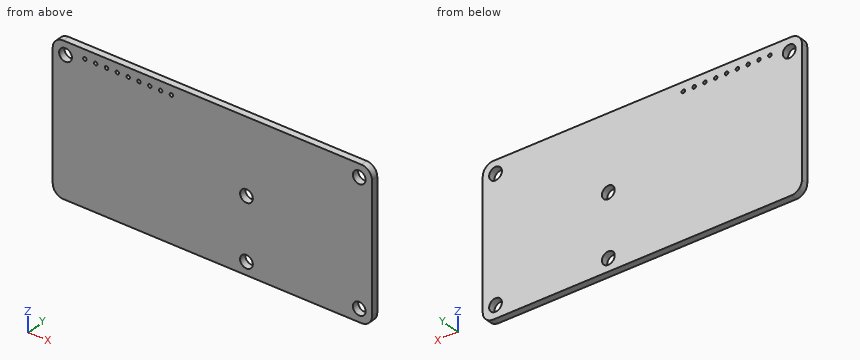
```python
from build123d import *

# Parameters (mm, degrees)
BOSS_EXTRUDE1_DEPTH = 1.6
SKETCH2_R           = 1.5
SKETCH2_R_2         = 0.406594982
CUT_EXTRUDE1_DEPTH  = 42.413282893


with BuildPart() as part:
    # Sketch1 → Boss-Extrude1 (new body)
    with BuildSketch(Plane(origin=(0, 0, 0), x_dir=(1, 0, 0), z_dir=(0, 1, 0))):
        with BuildLine():
            Line((-35, 17.5), (35, 17.5))
            ThreePointArc((35, 17.5), (36.767766953, 16.767766953), (37.5, 15))
            Line((37.5, 15), (37.5, -15))
            ThreePointArc((37.5, -15), (36.767766953, -16.767766953), (35, -17.5))
            Line((35, -17.5), (-35, -17.5))
            ThreePointArc((-35, -17.5), (-36.767766953, -16.767766953), (-37.5, -15))
            Line((-37.5, -15), (-37.5, 15))
            ThreePointArc((-37.5, 15), (-36.767766953, 16.767766953), (-35, 17.5))
        make_face()
    extrude(amount=BOSS_EXTRUDE1_DEPTH)

    # Sketch2 → Cut-Extrude1 (cut, through all)
    with BuildSketch(Plane(origin=(0, 1.6, 0), x_dir=(1, 0, 0), z_dir=(0, 1, 0))):
        with Locations(Location((-34.5, -14.5, 0), (0, 0, 270))):
            Circle(SKETCH2_R)
        with Locations(Location((34.5, -14.5, 0), (0, 0, 270))):
            Circle(SKETCH2_R)
        with Locations(Location((34.5, 14.5, 0), (0, 0, 270))):
            Circle(SKETCH2_R)
        with Locations(Location((8, 0, 0), (0, 0, 270))):
            Circle(SKETCH2_R)
        with Locations(Location((8, 14.5, 0), (0, 0, 270))):
            Circle(SKETCH2_R)
        with Locations(Location((-29.94018139, -15.399310559, 0), (0, 0, 270))):
            Circle(SKETCH2_R_2)
        with Locations(Location((-27.40018139, -15.399310559, 0), (0, 0, 270))):
            Circle(SKETCH2_R_2)
        with Locations(Location((-24.86018139, -15.399310559, 0), (0, 0, 270))):
            Circle(SKETCH2_R_2)
        with Locations(Location((-22.32018139, -15.399310559, 0), (0, 0, 270))):
            Circle(SKETCH2_R_2)
        with Locations(Location((-19.78018139, -15.399310559, 0), (0, 0, 270))):
            Circle(SKETCH2_R_2)
        with Locations(Location((-17.24018139, -15.399310559, 0), (0, 0, 270))):
            Circle(SKETCH2_R_2)
        with Locations(Location((-14.70018139, -15.399310559, 0), (0, 0, 270))):
            Circle(SKETCH2_R_2)
        with Locations(Location((-12.16018139, -15.399310559, 0), (0, 0, 270))):
            Circle(SKETCH2_R_2)
        with Locations(Location((-9.62018139, -15.399310559, 0), (0, 0, 270))):
            Circle(SKETCH2_R_2)
    extrude(amount=-CUT_EXTRUDE1_DEPTH, mode=Mode.SUBTRACT)


solid = part.part
```
Design review of the part built by this model. Coordinates are the model's own, in mm. Coordinates: 2 decimals unless noted, no trailing zeros. Order: outer loops, then holes, each group sorted by start corner. A loop starts at its lowest first (then second) coordinate and runs counter-clockwise, first axis right, second up. Notation, with made-up numbers: M -3.5,47 L 1.5,47 A12 ccw 1.5,69 Z; hole C 49.5,31.5 d7. An arc over 180 degrees is marked long. Answer as a JSON object with one key per item and string values. Group by question number.
1) Add section A-A, the plane z = 0. Write out the cut boundary in (x, y).
2) Add section B-B, the plane x = 8. Write out the cut boundary in (y, z), then the cut area to 3 significant figures.
3) For pin 1 (2.5 mm diameter, centred on x = 8, z = -14.5, fed in from -Y), flat-tipped, find the tip position at first contact; note if it passes through.
4) Wall thickness on L1, parallel to X at y = 0.55, z = -14.5; L2, parallel to X at y = 0.15, z = -13.5; L3, parallel to Z at x = -30, y = 0.3: over which ranges is each line inside the solid? List them lowest first.
5) Add section C-C, the plane y = 0.25. Count the separate pieces of the cut face and the enclosed holes in it, then the cut area to 3 significant figures.
Computed values:
{
 "1": {"outline": "M -37.5,0 L 6.5,0 L 6.5,1.6 L -37.5,1.6 Z; M 9.5,0 L 37.5,0 L 37.5,1.6 L 9.5,1.6 Z"},
 "2": {"outline": "M 0,-17.5 L 1.6,-17.5 L 1.6,-16 L 0,-16 Z; M 0,-13 L 1.6,-13 L 1.6,-1.5 L 0,-1.5 Z; M 0,1.5 L 1.6,1.5 L 1.6,17.5 L 0,17.5 Z", "area": "46.4 mm^2"},
 "3": {"pin 1": "passes through"},
 "4": {"L1": "x = -37.5 to 6.5, 9.5 to 33, 36 to 37.5", "L2": "x = -37.5 to 6.88, 9.12 to 33.38, 35.62 to 37.5", "L3": "z = -17.5 to 15, 15.8 to 17.5"},
 "5": {"separate pieces": "1", "enclosed holes": "14", "area": "2,580 mm^2"}
}
